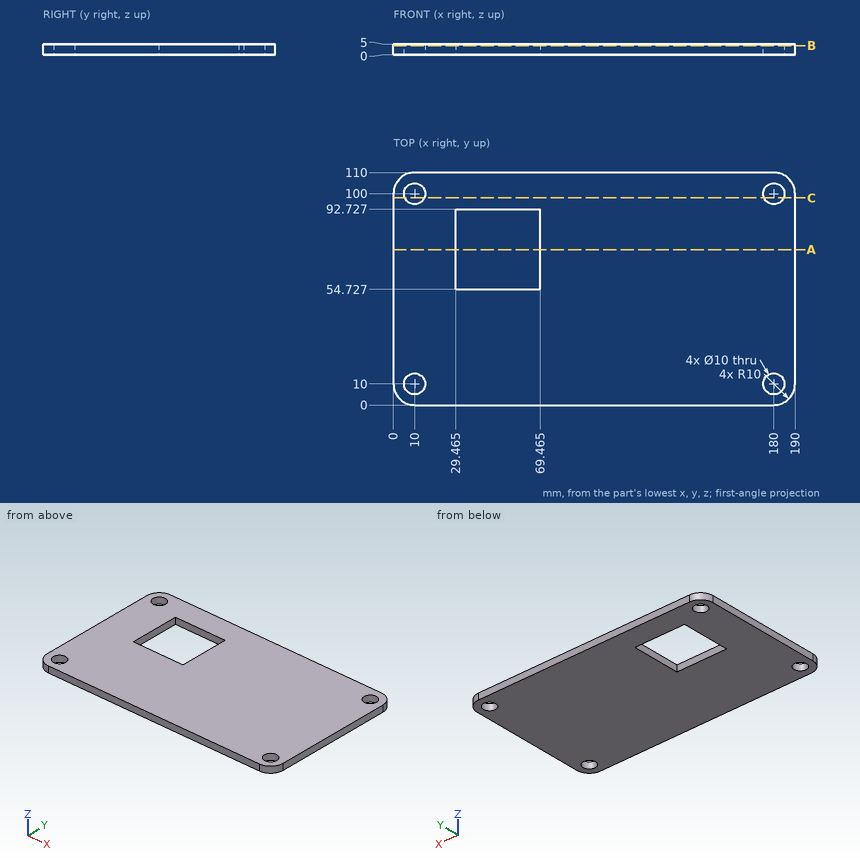
Design review of the part shown in the three views and the two pictorial views. Dimensions are in mm from the part's minimum x, y and z. Round coordinates to 2 decimals unless told otherwise and drop trailing zeros. Order: outer loops, then holes, each group sorted by start corner. A loop starts at its lowest first (then second) coordinate and runs counter-clockwise, first axis right, second up. Notation, with made-up numbers: (28.5, -5) -> (63.5, -5) arc R16 cw to (63.5, 3) -> close; hole circle Ø8 at (80.25, 9). An arc over 180 degrees is marked (long way). Write item = value, one per line. Start each with the question number.
1) Take a section at C-C on y = 98. State the section outline as (x, z) points.
2) Take a section at A-A on y = 73.5. State the section outline as (x, z) points (3 decimals).
3) To check wall thickness, follow line 1 (Y direction, x = 180, z = 2.4); line 2 (Y direction, x = 59, z = 2.3); line 3 (X direction, y = 86.5, z = 2.7) (3 decimals). State the ranges of each line that lie inside material, in increasing order. Write a range as from..to.
4) Take a section at B-B on z = 4.2. State the section outline as (x, y) points (3 decimals).
Verdict:
q1.outline = (0, 0) -> (5.42, 0) -> (5.42, 5) -> (0, 5) -> close; (14.58, 0) -> (175.42, 0) -> (175.42, 5) -> (14.58, 5) -> close; (184.58, 0) -> (190, 0) -> (190, 5) -> (184.58, 5) -> close
q2.outline = (0, 0) -> (29.465, 0) -> (29.465, 5) -> (0, 5) -> close; (69.465, 0) -> (190, 0) -> (190, 5) -> (69.465, 5) -> close
q3.line_1 = 0..5, 15..95, 105..110
q3.line_2 = 0..54.73, 92.73..110
q3.line_3 = 0..29.465, 69.465..190
q4.outline = (0, 10) arc R10 ccw to (10, 0) -> (180, 0) arc R10 ccw to (190, 10) -> (190, 100) arc R10 ccw to (180, 110) -> (10, 110) arc R10 ccw to (0, 100) -> close; hole circle Ø10 at (10, 10); hole circle Ø10 at (10, 100); hole (29.465, 54.727) -> (69.465, 54.727) -> (69.465, 92.727) -> (29.465, 92.727) -> close; hole circle Ø10 at (180, 10); hole circle Ø10 at (180, 100)
